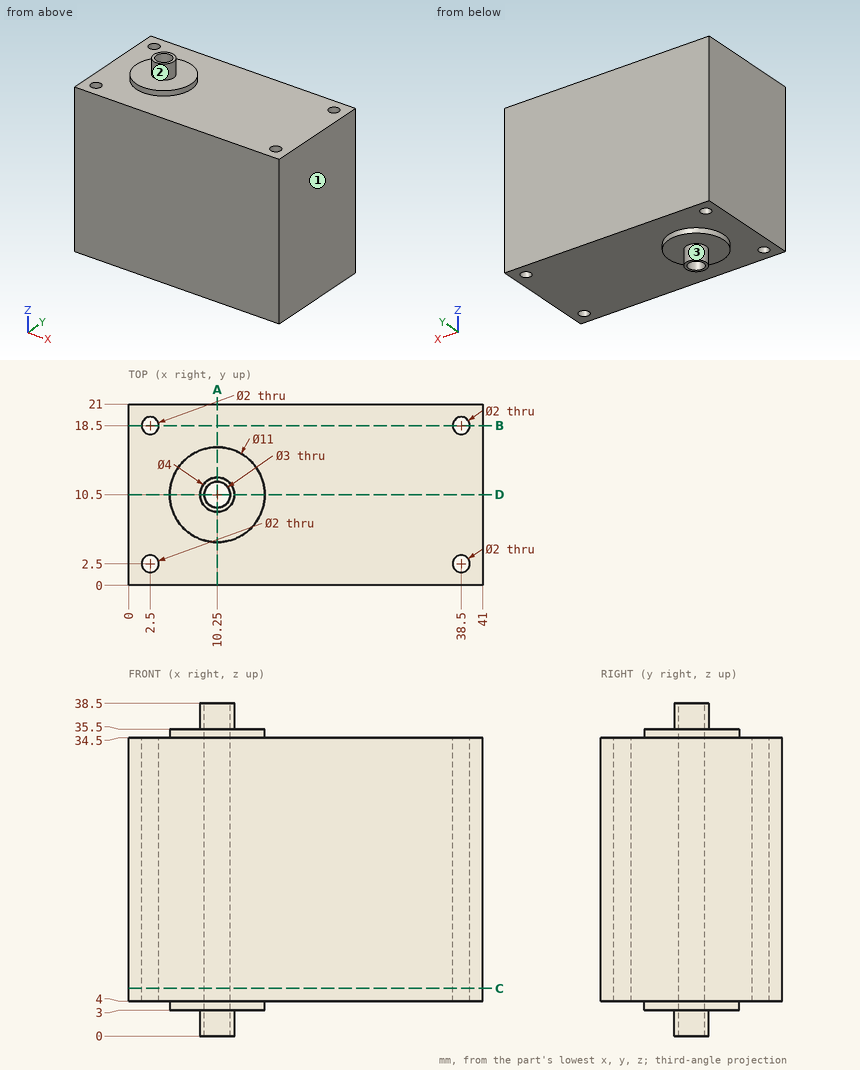
The drawing under review shows one solid part. Ordinate dimensions are in mm from its lowest x, y, z. A direction names the side the tool comes from. Round coordinates to 2 decimals unless told otherwise and drop trailing zeros. Write each loop counter-clockwise with the first axis right and the second up, starting at its lowest first coordinate (ties: lowest second). Pieces come first, ordered by that corner, then holes. Notation, with made-up numbers: (31.25, 37) - (67.25, 37) arc R32 ccw to (67.25, 75) - close; hole circle Ø2 at (20.25, 16.5). An arc over 180 degrees is marked (long way). Put each result on its own line as item: value.
Q1. We need section B-B (y = 18.5). Give the boundary of the cut face in (x, z), and give its area (3 significant figures).
Solved:
outline: (0, 4) - (1.5, 4) - (1.5, 34.5) - (0, 34.5) - close; (3.5, 4) - (37.5, 4) - (37.5, 34.5) - (3.5, 34.5) - close; (39.5, 4) - (41, 4) - (41, 34.5) - (39.5, 34.5) - close
area: 1,130 mm2
Q2. We need section A-A (x = 10.25). Give the boundary of the cut face in (y, z).
Solved:
outline: (0, 4) - (5, 4) - (5, 3) - (8.5, 3) - (8.5, 0) - (9, 0) - (9, 38.5) - (8.5, 38.5) - (8.5, 35.5) - (5, 35.5) - (5, 34.5) - (0, 34.5) - close; (12, 0) - (12.5, 0) - (12.5, 3) - (16, 3) - (16, 4) - (21, 4) - (21, 34.5) - (16, 34.5) - (16, 35.5) - (12.5, 35.5) - (12.5, 38.5) - (12, 38.5) - close
Q3. Wall thickness on probe 1 along X at (y, z) = (2.5, 29); probe 2 along Y at (x, z) = (2.5, 15); probe 3 along Y at (x, z) = (38, 10): over which ranges is each line inside the solid? List them lowest first.
Solved:
probe 1: x = 0 to 1.5, 3.5 to 37.5, 39.5 to 41
probe 2: y = 0 to 1.5, 3.5 to 17.5, 19.5 to 21
probe 3: y = 0 to 1.63, 3.37 to 17.63, 19.37 to 21
Q4. We need section C-C (z = 5.5). Give the boundary of the cut face in (x, y), and give its area (3 significant figures).
Solved:
outline: (0, 0) - (41, 0) - (41, 21) - (0, 21) - close; hole circle Ø2 at (2.5, 2.5); hole circle Ø2 at (2.5, 18.5); hole circle Ø3 at (10.25, 10.5); hole circle Ø2 at (38.5, 2.5); hole circle Ø2 at (38.5, 18.5)
area: 841 mm2
Q5. Machinability: for the marked faces 1, 2 and 3, which of the approach directions +Z, -Z, +X, -X, +Y, -Y give a long, thin tool a straight path to every point of the face, cutting with its end or side? Answer none if there is none.
Solved:
face 1: +Z, -Z, +X, +Y, -Y
face 2: +Z
face 3: -Z
Q6. We need section D-D (y = 10.5). Give the boundary of the cut face in (x, z), and give its area (3 significant figures).
Solved:
outline: (0, 4) - (4.75, 4) - (4.75, 3) - (8.25, 3) - (8.25, 0) - (8.75, 0) - (8.75, 38.5) - (8.25, 38.5) - (8.25, 35.5) - (4.75, 35.5) - (4.75, 34.5) - (0, 34.5) - close; (11.75, 0) - (12.25, 0) - (12.25, 3) - (15.75, 3) - (15.75, 4) - (41, 4) - (41, 34.5) - (15.75, 34.5) - (15.75, 35.5) - (12.25, 35.5) - (12.25, 38.5) - (11.75, 38.5) - close
area: 1,180 mm2
Q7. Insertion check: pin 1 Ø2 at (x, y) = (33, 11.5) entering from +Z; pin 2 Ø12 at (x, y) = (18, 2.5) entering from -Z. Each pin has a flat end and moves straight along its axis. Give the tip position at first contact, or say it passes through.
Solved:
pin 1: stops at z = 34.5
pin 2: stops at z = 3
